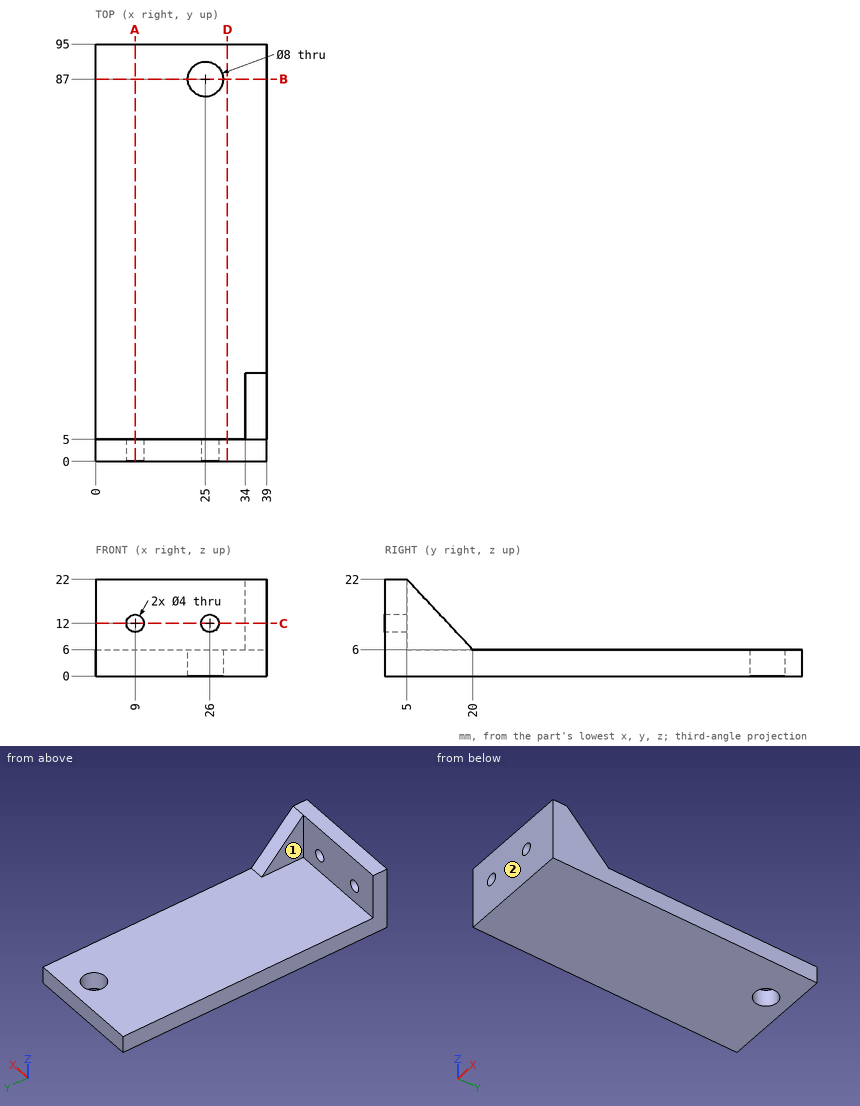
Design review of the part shown in the three views and the two pictorial views. Dimensions are in mm from the part's minimum x, y and z. A direction names the side the tool comes from. Round coordinates to 2 decimals unless told otherwise and drop trailing zeros. Write each loop counter-clockwise with the first axis right and the second up, starting at its lowest first coordinate (ties: lowest second). Pieces come first, ordered by that corner, then holes. Notation, with made-up numbers: (43, -33.75) -> (50, -33.75) arc R11 ccw to (50, -16.75) -> close; hole circle Ø6 at (53, 11.5). An arc over 180 degrees is marked (long way). Write item = value, one per line. Start each with the question number.
1) Wall thickness on probe 1 along X at (y, z) = (2.55, 12); probe 2 along Y at (x, z) = (25, 1.3); probe 3 along Z at (x, y) = (31.5, 31): over which ranges is each line inside the solid? List them lowest first. Write a range as from..to.
2) Take a section at B-B, the plane y = 87. State the section outline as (x, z) points, plus the area to 3 significant figures.
3) Take a section at A-A, the plane x = 9. State the section outline as (y, z) points, plus the area to 3 significant figures.
4) Take a section at C-C, the plane z = 12. State the section outline as (x, y) points (3 decimals), plus the area to 3 significant figures.
5) Tool access review of the marked faces 1 and 2: name each direction out of +Z, -Z, +X, -X, +Y, -Y from which nothing blocks a thin tool from reaching the whole face with its end or side.
6) Take a section at D-D, the plane x = 30. State the section outline as (y, z) points.
7) Clearance check with flat-ended pins moving along their axes: pin 1 (4.5 mm diameter, centred on y = 10.5, z = 13.5, fed in from -X); pin 2 (2 mm diameter, centred on x = 18.5, z = 18, fed in from +Y); pin 3 (8 mm diameter, centred on x = 22, y = 18, fed in from +Z). State where each tip first meets the part, or that it passes through.
Results list:
q1.probe_1 = 0..7, 11..24, 28..39
q1.probe_2 = 0..83, 91..95
q1.probe_3 = 0..6
q2.outline = (0, 0) -> (21, 0) -> (21, 6) -> (0, 6) -> close; (29, 0) -> (39, 0) -> (39, 6) -> (29, 6) -> close
q2.area = 186 mm²
q3.outline = (0, 0) -> (95, 0) -> (95, 6) -> (5, 6) -> (5, 10) -> (0, 10) -> close; (0, 14) -> (5, 14) -> (5, 22) -> (0, 22) -> close
q3.area = 630 mm²
q4.outline = (0, 0) -> (7, 0) -> (7, 5) -> (0, 5) -> close; (11, 0) -> (24, 0) -> (24, 5) -> (11, 5) -> close; (28, 0) -> (39, 0) -> (39, 14.375) -> (34, 14.375) -> (34, 5) -> (28, 5) -> close
q4.area = 202 mm²
q5.face_1 = +Z, -X, +Y
q5.face_2 = +Z, -Z, +X, -X, -Y
q6.outline = (0, 0) -> (95, 0) -> (95, 6) -> (5, 6) -> (5, 22) -> (0, 22) -> close
q7.pin_1 = 34
q7.pin_2 = 5
q7.pin_3 = 6
